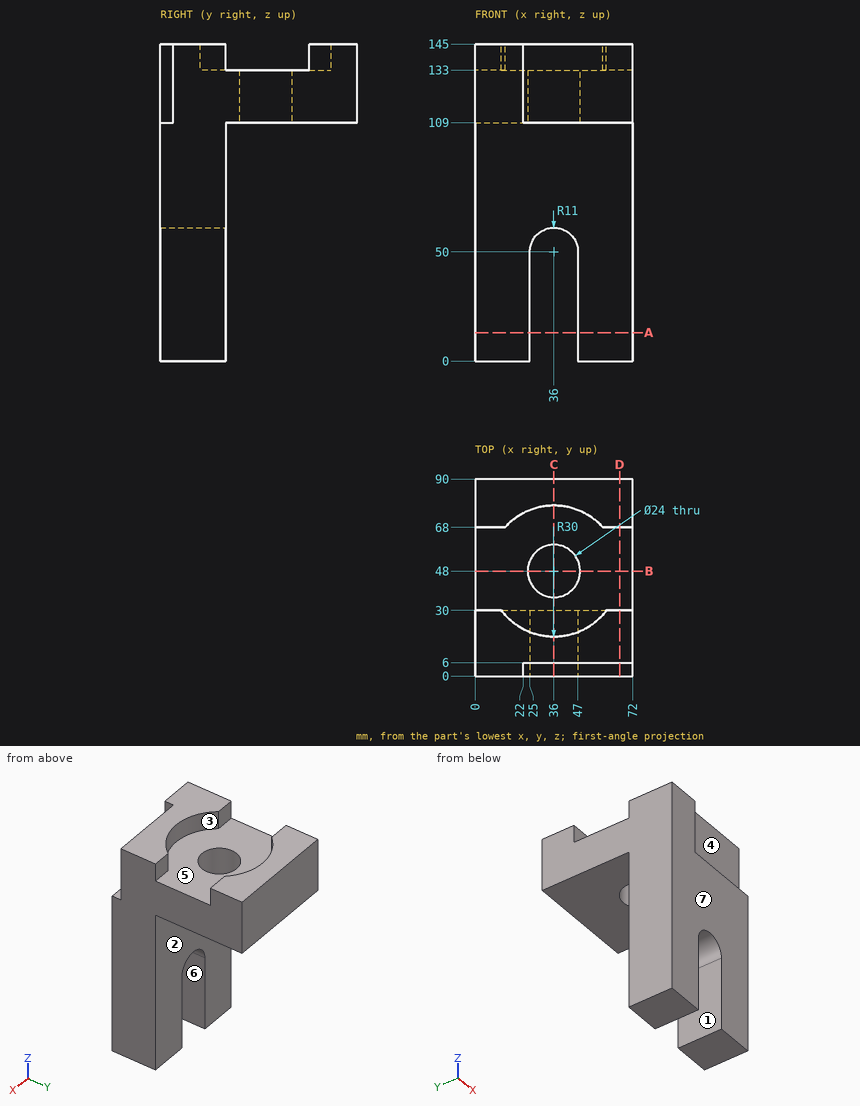
Source: three-view drawing plus pictorial views. Frame: mm from the lowest corner of the part. A direction names the side the tool comes from. Coordinates: 2 decimals unless noted, no trailing zeros. Loops run counter-clockwise (first coordinate to the right, second up) from the corner with the lowest first, then second, coordinate; pieces in that order, holes last. Notation, with made-up numbers: (12, 68.5) -> (54, 68.5) arc R12 ccw to (54, 77.5) -> close; hole circle Ø3 at (49.25, 32.5). An arc over 180 degrees is marked (long way). One line per item, written item: value.
(1) Set-up query: the marked faces 1, 2, 3 and 4. Return all of +Z, -Z, +X, -X, +Y, -Y with unobstructed straight access to the full face (end or side cutting, diameter ignored); none if empty.
Answer below:
face 1: -Z, +Y, -Y
face 2: -Z, +X, -X, +Y
face 3: +Z
face 4: +Z, +X, -Y
(2) Cut plane B-B (y = 48). Output: boundary loops of the cut face in (x, z).
Answer below:
outline: (0, 109) -> (24, 109) -> (24, 133) -> (0, 133) -> close; (48, 109) -> (72, 109) -> (72, 133) -> (48, 133) -> close
(3) Ray query, line 1 along Y through (x, z) = (36, 118.5); line 2 along Y through (x, z) = (11, 95); line 3 along Z through (x, y) = (19.5, 68). Return the intervals inside material, ascending.
Answer below:
line 1: y = 6 to 36, 60 to 90
line 2: y = 0 to 30
line 3: z = 109 to 133
(4) Draft query along Y for the marked faces 5, 6 and 7. Return one class per face: pulls with the +Y half, pulls with the -Y half, needs draft (parallel to the pull), parting line crosses it, or undercut.
Answer below:
face 5: undercut
face 6: needs draft
face 7: pulls with the -Y half
(5) Cut plane A-A (z = 13). Output: boundary loops of the cut face in (x, y), then the cut area to 3 significant figures.
Answer below:
outline: (0, 0) -> (25, 0) -> (25, 30) -> (0, 30) -> close; (47, 0) -> (72, 0) -> (72, 30) -> (47, 30) -> close
area: 1,500 mm2
(6) Cut plane C-C (x = 36). Output: boundary loops of the cut face in (y, z), then the cut area to 3 significant figures.
Answer below:
outline: (0, 61) -> (30, 61) -> (30, 109) -> (36, 109) -> (36, 133) -> (18, 133) -> (18, 145) -> (6, 145) -> (6, 109) -> (0, 109) -> close; (60, 109) -> (90, 109) -> (90, 145) -> (78, 145) -> (78, 133) -> (60, 133) -> close
area: 3,170 mm2
(7) Cut plane D-D (x = 66). Output: boundary loops of the cut face in (y, z), then the cut area to 3 significant figures.
Answer below:
outline: (0, 0) -> (30, 0) -> (30, 109) -> (90, 109) -> (90, 145) -> (68, 145) -> (68, 133) -> (30, 133) -> (30, 145) -> (6, 145) -> (6, 109) -> (0, 109) -> close
area: 5,840 mm2
(8) Pin query (flat end, axial travel): pin 1 Ø10 at (x, y) = (46, 42.5) entering from -Z; pin 2 Ø1.8 at (y, z) = (1.5, 129.5) entering from +X; pin 3 Ø18 at (x, y) = (30, 43) entering from +Z; pin 4 Ø12 at (x, z) = (36.5, 16.5) entering from +Y. Return the tip coordinate at first contact, or that it passes through.
Answer below:
pin 1: stops at z = 109
pin 2: stops at x = 22
pin 3: stops at z = 133
pin 4: passes through
